```python
from build123d import *

# Parameters (mm, degrees)
F1_DEPTH = 8.89
F2_T     = -2.54
F4_DEPTH = 2.54


with BuildPart() as f1:
    # F0 (on Front) → F1 (new body, symmetric)
    with BuildSketch(Plane.XZ):
        Polygon((-12.7, -279.4), (0, -279.4), (0, 0), (342.9, 0), (342.9, -279.4), (355.6, -279.4), (355.6, 12.7), (-12.7, 12.7), align=None)
    extrude(amount=F1_DEPTH, both=True)

    # F2
    f2_openings = [f1.faces().sort_by_distance(p)[0] for p in [
        (171.45, 0, 0),
        (0, 0, -139.7),
        (-6.35, 0, -279.4),
        (342.9, 0, -139.7),
        (349.25, 0, -279.4),
    ]]
    offset(amount=F2_T, openings=f2_openings)

    # F3 (on face) → F4 (join)
    with BuildSketch(Plane(origin=(0, 8.89, 0), x_dir=(-1, 0, 0), z_dir=(0, 1, 0))):
        Polygon((-381, 38.1), (-381, -330.2), (-342.9, -330.2), (-342.9, -279.4), (-355.6, -279.4), (-355.6, 12.7), (12.7, 12.7), (12.7, -279.4), (0, -279.4), (0, -330.2), (38.1, -330.2), (38.1, 38.1), align=None)
    extrude(amount=-F4_DEPTH)


solid = f1.part
```
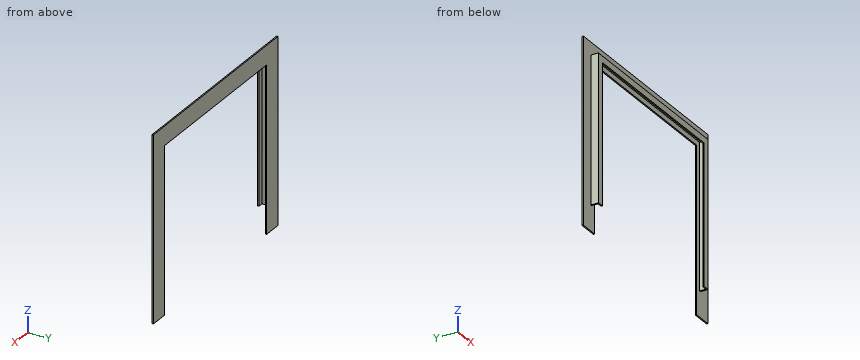
The listing builds one solid part. Answer for the finished solid, in the listing's coordinates (mm). Round coordinates to 2 decimals unless told otherwise and drop trailing zeros. Loops run counter-clockwise (first coordinate to the right, second up) from the corner with the lowest first, then second, coordinate; pieces in that order, holes last.
1) A cutting plane is placed at A-A on z = -137. Determine the outline of the cut face in (x, y), plus the area to 3 significant figures.
Outcome:
outline: (-38.1, 6.35) - (-12.7, 6.35) - (-12.7, -8.89) - (0, -8.89) - (0, -6.35) - (-10.16, -6.35) - (-10.16, 6.35) - (0, 6.35) - (0, 8.89) - (-38.1, 8.89) - close; (342.9, -8.89) - (355.6, -8.89) - (355.6, 6.35) - (381, 6.35) - (381, 8.89) - (342.9, 8.89) - (342.9, 6.35) - (353.06, 6.35) - (353.06, -6.35) - (342.9, -6.35) - close
area: 323 mm2
2) A cutting plane is placed at B-B on y = -1.5. Determine the outline of the cut face in (x, z), plus the area to 3 significant figures.
Outcome:
outline: (-12.7, -279.4) - (-10.16, -279.4) - (-10.16, 10.16) - (353.06, 10.16) - (353.06, -279.4) - (355.6, -279.4) - (355.6, 12.7) - (-12.7, 12.7) - close
area: 2,410 mm2
3) Consider line 1 (X direction, y = 5.5, z = 2.5); line 2 (X direction, y = -7, z = -122); line 3 (Z direction, x = 295.5, y = 7.5). Determine where each line is inside the solid, lowest interval first.
Outcome:
line 1: x = -12.7 to -10.16, 353.06 to 355.6
line 2: x = -12.7 to 0, 342.9 to 355.6
line 3: z = 0 to 38.1
4) A cutting plane is placed at C-C on x = 161. Determine the outline of the cut face in (y, z), plus the area to 3 significant figures.
Outcome:
outline: (-8.89, 0) - (-6.35, 0) - (-6.35, 10.16) - (6.35, 10.16) - (6.35, 0) - (8.89, 0) - (8.89, 38.1) - (6.35, 38.1) - (6.35, 12.7) - (-8.89, 12.7) - close
area: 161 mm2
5) Given P1, Ø5, axis at x = 82, y = 6, coming from the -Z side; P2, Ø1.3, axis at y = -7.5, z = -134, coming from the -X side; P3, Ø0.8, axis at y = -7, z = -98, coming from the +X side, each flat-ended and moving along its own axis, determine where each tip first touches the part or whether it passes through.
Outcome:
P1: stops at z = 0
P2: stops at x = -12.7
P3: stops at x = 355.6
